The model under review builds one solid part; all positions refer to its coordinate system, in mm. A direction names the side the tool comes from. Round coordinates to 2 decimals unless told otherwise and drop trailing zeros. Write each loop counter-clockwise with the first axis right and the second up, starting at its lowest first coordinate (ties: lowest second). Pieces come first, ordered by that corner, then holes. Notation, with made-up numbers: (-31, 6.5) - (1, 6.5) arc R25 ccw to (1, 36.5) - close; hole circle Ø3 at (-33, 37). An arc over 180 degrees is marked (long way). Return JSON: item names as keys, results as strings.
from build123d import *

# Parameters (mm, degrees)
BOSS_EXTRUDE1_DEPTH = 38.1
SKETCH2_R           = 0.762
CUT_EXTRUDE1_DEPTH  = 7.62
CUT_EXTRUDE2_START  = -7.62
SKETCH3_R           = 0.762
CUT_EXTRUDE2_DEPTH  = 7.62


with BuildPart() as part:
    # Sketch1 → Boss-Extrude1 (new body)
    with BuildSketch(Plane.XY):
        Polygon((0, 0), (7.112, 0), (4.571451506, 5.08), (-2.540548494, 5.08), align=None)
    extrude(amount=-BOSS_EXTRUDE1_DEPTH)

    # Sketch2 → Cut-Extrude1 (cut)
    with BuildSketch(Plane.XY):
        with Locations((1.979121083, 2.54)):
            Circle(SKETCH2_R)
    extrude(amount=-CUT_EXTRUDE1_DEPTH, mode=Mode.SUBTRACT)

    # Sketch3 → Cut-Extrude2 (cut)
    with BuildSketch(Plane(origin=(0, 0, -38.1), x_dir=(-1, 0, 0), z_dir=(0, 0, -1)).offset(CUT_EXTRUDE2_START)):
        with Locations(Location((-1.979121083, 2.54, 0), (0, 0, 180))):
            Circle(SKETCH3_R)
    extrude(amount=CUT_EXTRUDE2_DEPTH, mode=Mode.SUBTRACT)


solid = part.part
(1) Wall thickness on line 1 (Y direction, x = 2, z = -33.5); line 2 (X direction, y = 2.54, z = -35); line 3 (Y direction, x = -0.75, z = -19): over which ranges is each line inside the solid? List them lowest first.
Filled in:
{"line 1": "y = 0 to 1.78, 3.3 to 5.08", "line 2": "x = -1.27 to 1.22, 2.74 to 5.84", "line 3": "y = 1.5 to 5.08"}
(2) Add section C-C (x = 1.75). Write out the cut boundary in (y, z), plus the area to 3 significant figures.
Filled in:
{"outline": "(0, -38.1) - (1.81, -38.1) - (1.81, -30.48) - (3.27, -30.48) - (3.27, -38.1) - (5.08, -38.1) - (5.08, 0) - (3.27, 0) - (3.27, -7.62) - (1.81, -7.62) - (1.81, 0) - (0, 0) - close", "area": "171 mm2"}
(3) Add section A-A (z = -3). Write out the cut boundary in (x, y).
Filled in:
{"outline": "(-2.54, 5.08) - (0, 0) - (7.11, 0) - (4.57, 5.08) - close; hole circle Ø1.52 at (1.98, 2.54)"}
(4) Clearance check with flat-ended pins moving along their axes: pin 1 Ø1.5 at (y, z) = (2.5, -13.5) entering from +X; pin 2 Ø1 at (y, z) = (3, -12.5) entering from +X; pin 3 Ø2 at (y, z) = (3, -26.5) entering from +X. State where each tip first meets the part, or that it passes through.
Filled in:
{"pin 1": "stops at x = 6.24", "pin 2": "stops at x = 5.86", "pin 3": "stops at x = 6.11"}
(5) For faces 4 (the cylindrical face through (1.8, 1.8, -3.8)), 5 (the flat face through (5.86, 2.5, -18.78)), 6 (the flat face through (2, 3, -30.48)), list the 3-axis set-ups (+Z, -Z, +X, -X, +Y, -Y) from which the entire face can be reached by the end or side of a thin tool; tool diameter is ignored.
Filled in:
{"face 4": "+Z", "face 5": "+Z, -Z, +X, +Y", "face 6": "-Z"}
(6) Add section B-B (z = -18.5). Write out the cut boundary in (x, y), plus the area to 3 significant figures.
Filled in:
{"outline": "(-2.54, 5.08) - (0, 0) - (7.11, 0) - (4.57, 5.08) - close", "area": "36.1 mm2"}
(7) Add section D-D (y = 2.54). Write out the cut boundary in (x, z).
Filled in:
{"outline": "(-1.27, -38.1) - (1.22, -38.1) - (1.22, -30.48) - (2.74, -30.48) - (2.74, -38.1) - (5.84, -38.1) - (5.84, 0) - (2.74, 0) - (2.74, -7.62) - (1.22, -7.62) - (1.22, 0) - (-1.27, 0) - close"}
(8) Mouldability with a two-part tool opening along X and no side actions: class faces 1 (the flat face through (-1.3, 2.6, -18.8)), 2 (the flat face through (2, 3, -7.62)), 3 (the flat face through (1, 3, -38.1)) as released by +X, released by -X, zero draft, split by the parting line, or undercut.
Filled in:
{"face 1": "released by -X", "face 2": "undercut", "face 3": "zero draft"}
